```python
from build123d import *

# Parameters (mm, degrees)
SKETCH2_W = 70.25
SKETCH2_H = 21.6


with BuildPart() as part:
    # Sweep1: sweep along a curve in space
    with BuildLine() as sweep1_path:
        Line((3251.181818755, -307.327166096, 1441.624252092), (3251.181818755, -307.327166096, 1381.624252092))
        Line((3215.675, 0, 1165), (3251.181818755, -307.327166096, 1381.624252092))
        Line((3215.675, 0, 1165), (3215.675, 0, 0))
        Line((3215.675, 0, 0), (3247.785290657, 341.355989282, -240.075201436))
        Line((3247.785290657, 341.355989282, -240.075201436), (3247.785290657, 341.355989282, -300.075201436))
    # Sketch2 → Sweep1 (sweep)
    with BuildSketch(Plane(origin=(3247.785290657, 341.355989282, -300.075201436), x_dir=(1, 0, 0), z_dir=(0, 0, 1))):
        Rectangle(SKETCH2_W, SKETCH2_H)
    sweep(path=sweep1_path.line, transition=Transition.RIGHT)


solid = part.part
```
Input: part model. Units: mm. Frame: model coordinates. A direction names the side the tool comes from. Give positions to 0.01 mm unless a question says otherwise; leave off trailing zeros. Order: outer loops, then holes, each group sorted by start corner. A loop starts at its lowest first (then second) coordinate and runs counter-clockwise, first axis right, second up. Notation, with made-up numbers: (73.5, -15.5) - (83.5, -15.5) arc R18 cw to (83.5, 6.5) - close; hole circle Ø7 at (-16, -5). An arc over 180 degrees is marked (long way). Use a Markdown table: item, result.
(1) Section query B-B (y = 171.5). Output: boundary loops of the cut face in (x, z), then the cut area to 3 significant figures.
Computed values:
| item | result |
|---|---|
| outline | (3195.67, -109.14) - (3197.7, -135.52) - (3267.95, -132.1) - (3265.92, -105.71) - close |
| area | 1,860 mm2 |
(2) Access query for faces 1 (the flat face through (3216, 10.8, 580)), 2 (the flat face through (3215, -10.8, 569)), 3 (the flat face through (3233, -162, 1266)). Directions: +Z, -Z, +X, -X, +Y, -Y. A direction counts if a zero-diameter tool reaches every point of the face in a straight line with its end or side. Return the directions, or none.
Computed values:
| item | result |
|---|---|
| face 1 | +Z, +X, -X, +Y |
| face 2 | -Z, +X, -X, -Y |
| face 3 | -Z, -X, -Y |
(3) Pin query (flat end, axial travel): pin 1 (6 mm diameter, centred on x = 3225.5, z = 817.5, fed in from +Y); pin 2 (24 mm diameter, centred on y = 345, z = -258, fed in from -X); pin 3 (4 mm diameter, centred on x = 3198.5, y = -54.5, fed in from +Z). Return the tip coordinate at first contact, or that it passes through.
Computed values:
| item | result |
|---|---|
| pin 1 | stops at y = 10.8 |
| pin 2 | stops at x = 3212.66 |
| pin 3 | stops at z = 1219.52 |
(4) Section query A-A (z = 525.5). Output: boundary loops of the cut face in (x, y), then the cut area to 3 significant figures.
Computed values:
| item | result |
|---|---|
| outline | (3180.55, -10.8) - (3250.8, -10.8) - (3250.8, 10.8) - (3180.55, 10.8) - close |
| area | 1,520 mm2 |
(5) Line query: line 1 (Y direction, x = 3202.5, z = 498); line 2 (Z direction, x = 3219.5, y = -14.5); line 3 (Z direction, x = 3231.5, y = 108). Output: solid intervals per line, ascending. Write a range as from..to.
Computed values:
| item | result |
|---|---|
| line 1 | y = -10.8..10.8 |
| line 2 | z = 1161.82..1188.36 |
| line 3 | z = -88.92..-62.44 |
